from build123d import *

# Parameters (mm, degrees)
BOSS_EXTRUDE1_DEPTH = 25.4
SKETCH2_R           = 3.302
CUT_EXTRUDE1_DEPTH  = 25.4
FILLET1_R           = 0.508
FILLET2_R           = 0.254
FILLET3_R           = 2
FILLET4_R           = 4
FILLET5_R           = 0.5


with BuildPart() as part:
    # Sketch1 → Boss-Extrude1 (new body)
    with BuildSketch(Plane(origin=(0, 0, 0), x_dir=(1, 0, 0), z_dir=(0, 1, 0))):
        with BuildLine():
            Line((-13.248638633, -3.549962023), (-12.021912834, -3.221261835))
            ThreePointArc((-12.021912834, -3.221261835), (0, 12.446), (12.021912834, -3.221261835))
            Line((12.021912834, -3.221261835), (13.248638633, -3.549962023))
            ThreePointArc((13.248638633, -3.549962023), (12.968835743, 4.465193777), (8.255, 10.953703985))
            Line((8.255, 10.953703985), (8.255, 14.716))
            Line((8.255, 14.716), (8.255, 21.701))
            Line((8.255, 21.701), (-8.255, 21.701))
            Line((-8.255, 21.701), (-8.255, 14.716))
            Line((-8.255, 14.716), (-8.255, 10.953703985))
            ThreePointArc((-8.255, 10.953703985), (-12.968835743, 4.465193777), (-13.248638633, -3.549962023))
        make_face()
    extrude(amount=BOSS_EXTRUDE1_DEPTH)

    # Sketch2 → Cut-Extrude1 (cut)
    with BuildSketch(Plane(origin=(0, 25.4, 0), x_dir=(1, 0, 0), z_dir=(0, 1, 0))):
        with Locations((0, 19.28817272)):
            Circle(SKETCH2_R)
        with BuildLine():
            Line((-8.255, 21.701), (-8.255, 14.716))
            add(Edge.make_bspline(
                [(-8.255, 14.716), (-4.739338783, 15.636189596), (-6.519245554, 19.893117267), (-4.063143766, 21.701)],
                knots=[0, 0, 0, 0, 1, 1, 1, 1], degree=3))
            Line((-4.063143766, 21.701), (-8.255, 21.701))
        make_face()
        with BuildLine():
            Line((8.255, 21.701), (8.255, 14.716))
            add(Edge.make_bspline(
                [(8.255, 14.716), (4.739338783, 15.636189596), (6.519245554, 19.893117267), (4.063143766, 21.701)],
                knots=[0, 0, 0, 0, 1, 1, 1, 1], degree=3))
            Line((4.063143766, 21.701), (8.255, 21.701))
        make_face()
    extrude(amount=-CUT_EXTRUDE1_DEPTH, mode=Mode.SUBTRACT)

    # Fillet1
    fillet1_edges = [part.edges().sort_by_distance(p)[0] for p in [
        (-4.063143766, 12.7, -21.701),
        (4.063143766, 12.7, -21.701),
    ]]
    fillet(fillet1_edges, radius=FILLET1_R)

    # Fillet2
    fillet2_edges = [part.edges().sort_by_distance(p)[0] for p in [
        (2.254211285, 12.7, -21.701),
        (-2.254211285, 12.7, -21.701),
    ]]
    fillet(fillet2_edges, radius=FILLET2_R)

    # Fillet3
    fillet3_edges = [part.edges().sort_by_distance(p)[0] for p in [
        (-8.255, 12.7, -14.716),
        (8.255, 12.7, -14.716),
    ]]
    fillet(fillet3_edges, radius=FILLET3_R)

    # Fillet4
    fillet4_edges = [part.edges().sort_by_distance(p)[0] for p in [
        (-8.255, 12.7, -10.953703985),
        (8.255, 12.7, -10.953703985),
    ]]
    fillet(fillet4_edges, radius=FILLET4_R)

    # Fillet5
    fillet5_edges = [part.edges().sort_by_distance(p)[0] for p in [
        (13.248638633, 12.7, 3.549962023),
        (12.021912834, 12.7, 3.221261835),
        (-12.021912834, 12.7, 3.221261835),
        (-13.248638633, 12.7, 3.549962023),
    ]]
    fillet(fillet5_edges, radius=FILLET5_R)


solid = part.part
Part model, mm, in its own coordinate system. Round coordinates to 2 decimals unless told otherwise and drop trailing zeros. Order: outer loops, then holes, each group sorted by start corner. A loop starts at its lowest first (then second) coordinate and runs counter-clockwise, first axis right, second up. Notation, with made-up numbers: (71.25, 31) -> (128.25, 31) arc R25 ccw to (128.25, 43) -> close; hole circle Ø8 at (36.25, 59). An arc over 180 degrees is marked (long way). Put each result on its own line as item: value.
Q1. Pin check, flat tips, straight feed: pin 1 Ø10 at (x, z) = (-1, -5.5) entering from +Y; pin 2 Ø4 at (y, z) = (13, -8) entering from +X; pin 3 Ø0.7 at (y, z) = (7, -13) entering from -X. Stop position of each tip, or through.
From the geometry:
pin 1: passes through
pin 2: stops at x = 12.33
pin 3: stops at x = -8.26
Q2. Band-saw the part on C-C (z = -3.25). Give the cut face in (x, y), and give its area (3 significant figures).
From the geometry:
outline: (-13.33, 0) -> (-12.01, 0) -> (-12.01, 25.4) -> (-13.33, 25.4) -> close; (12.01, 0) -> (13.33, 0) -> (13.33, 25.4) -> (12.01, 25.4) -> close
area: 66.6 mm2
Q3. Band-saw the part on A-A (z = 0). Give the cut face in (x, y), and give its area (3 significant figures).
From the geometry:
outline: (-13.72, 0) -> (-12.45, 0) -> (-12.45, 25.4) -> (-13.72, 25.4) -> close; (12.45, 0) -> (13.72, 0) -> (13.72, 25.4) -> (12.45, 25.4) -> close
area: 64.5 mm2
Q4. Band-saw the part on B-B (x = 0). Give the cut face in (y, z).
From the geometry:
outline: (0, -15.99) -> (25.4, -15.99) -> (25.4, -12.45) -> (0, -12.45) -> close
Q5. Band-saw the part on D-D (x = 10.5). Give the cut face in (y, z), and give its area (3 significant figures).
From the geometry:
outline: (0, -8.82) -> (25.4, -8.82) -> (25.4, -6.68) -> (0, -6.68) -> close
area: 54.4 mm2
Q6. Pull direction X, two halves, no side cores. Call faces 1 (the face through (0, 0, -13)), 2 (the face through (13.166, 12.522, -3.846)), 3 (the face through (-0.103, 12.878, -15.988)): pulls with the +X half, pulls with the -X half, needs draft (parallel to the pull), parting line crosses it, or undercut.
From the geometry:
face 1: needs draft
face 2: pulls with the +X half
face 3: undercut
Q7. Wall check: line 1 (X direction, y = 9.5, z = 0); line 2 (Z direction, x = 0, y = 14.75); line 3 (X direction, y = 16, z = -4.75). Give the ranges that are in metal, low to high. Write a range as [from, to].
From the geometry:
line 1: x = [-13.72, -12.45], [12.45, 13.72]
line 2: z = [-15.99, -12.45]
line 3: x = [-12.87, -11.5], [11.5, 12.87]
